from build123d import *

# Parameters (mm, degrees)
F1_DEPTH = 60
F3_D     = 4
F4_D     = 4.5
F5_D     = 5
F6_D     = 5.5
F7_D     = 6
F8_R     = 5.08


with BuildPart() as f1:
    # F0 (on Top) → F1 (new body)
    with BuildSketch(Plane.XY):
        Polygon((-18.362068, 0), (-17.327586, 0), (16.637932, 0), (16.637932, 38.40517), (6.637932, 38.40517), (6.637932, 15), (-8.362068, 15), (-8.362068, 38.40517), (-18.362068, 38.40517), align=None)
    extrude(amount=F1_DEPTH)

    # F3 (through all)
    with Locations(Plane.XZ):
        with Locations((-0.862068, 10)):
            Hole(F3_D / 2)

    # F4 (through all)
    with Locations(Plane.XZ):
        with Locations((-0.862068, 20)):
            Hole(F4_D / 2)

    # F5 (through all)
    with Locations(Plane.XZ):
        with Locations((-0.862068, 30)):
            Hole(F5_D / 2)

    # F6 (through all)
    with Locations(Plane.XZ):
        with Locations((-0.862068, 40)):
            Hole(F6_D / 2)

    # F7 (through all)
    with Locations(Plane.XZ):
        with Locations((-0.862068, 50)):
            Hole(F7_D / 2)

    # F8
    f8_edges = [f1.edges().sort_by_distance(p)[0] for p in [
        (16.637932, 0, 30),
        (-0.862068, 0, 60),
        (-18.362068, 0, 30),
        (-0.862068, 0, 0),
        (-18.362068, 19.202585, 60),
        (16.637932, 19.202585, 60),
        (-18.362068, 19.202585, 0),
        (16.637932, 19.202585, 0),
    ]]
    fillet(f8_edges, radius=F8_R)


solid = f1.part
Part model, mm, in its own coordinate system. A direction names the side the tool comes from. Coordinates: 2 decimals unless noted, no trailing zeros. Order: outer loops, then holes, each group sorted by start corner. A loop starts at its lowest first (then second) coordinate and runs counter-clockwise, first axis right, second up. Notation, with made-up numbers: M -8.75,28 L 22.25,28 A23 ccw 22.25,57 Z; hole C -19,56 d9. An arc over 180 degrees is marked long. One line per question, with ' | ' between items.
Q1. Slice it at A-A (z = 30). Give the cut face in (x, y), and give its area (3 significant figures).
A:
outline: M -18.36,5.08 A5.08 ccw -13.28,0 L -3.36,0 L -3.36,15 L -8.36,15 L -8.36,38.41 L -18.36,38.41 Z; M 1.64,0 L 11.56,0 A5.08 ccw 16.64,5.08 L 16.64,38.41 L 6.64,38.41 L 6.64,15 L 1.64,15 Z | area: 907 mm^2
Q2. Slice it at C-C (x = -0.5). Give the cut face in (y, z), and give its area (3 significant figures).
A:
outline: M 0,5.08 A5.08 ccw 5.08,0 L 15,0 L 15,8.03 L 0,8.03 Z; M 0,11.97 L 15,11.97 L 15,17.78 L 0,17.78 Z; M 0,22.22 L 15,22.22 L 15,27.53 L 0,27.53 Z; M 0,32.47 L 15,32.47 L 15,37.27 L 0,37.27 Z; M 0,42.73 L 15,42.73 L 15,47.02 L 0,47.02 Z; M 0,52.98 L 15,52.98 L 15,60 L 5.08,60 A5.08 ccw 0,54.92 Z | area: 518 mm^2
Q3. Slice it at B-B (y = 28.5). Give the cut face in (x, z), and give its area (3 significant figures).
A:
outline: M -18.36,5.08 A5.08 ccw -13.28,0 L -8.36,0 L -8.36,60 L -13.28,60 A5.08 ccw -18.36,54.92 Z; M 6.64,0 L 11.56,0 A5.08 ccw 16.64,5.08 L 16.64,54.92 A5.08 ccw 11.56,60 L 6.64,60 Z | area: 1,180 mm^2
Q4. Slice it at D-D (y = 13.5). Give the cut face in (x, z).
A:
outline: M -18.36,5.08 A5.08 ccw -13.28,0 L 11.56,0 A5.08 ccw 16.64,5.08 L 16.64,54.92 A5.08 ccw 11.56,60 L -13.28,60 A5.08 ccw -18.36,54.92 Z; hole C -0.86,50 d6; hole C -0.86,40 d5.5; hole C -0.86,30 d5; hole C -0.86,20 d4.5; hole C -0.86,10 d4
Q5. Two-plate mould, pull along Z, no slides. Class faces 3 (the face through (-1, 14.6, 60)), 4 (the face through (-16.913, 21.509, 1.528)), 5 (the face through (-0.504, 7.605, 42.727)): +Z half, -Z half, draft (parallel to the pull), parting line (faces both ways), or undercut.
A:
face 3: +Z half | face 4: -Z half | face 5: undercut
Q6. 3-axis set-ups, long thin cutter, end or side, ignore diameter. For faces 1 (the face through (15.11, 21.98, 58.55)), 2 (the face through (3, 15, 30)): which of +Z, -Z, +X, -X, +Y, -Y reach the whole face in a straight line?
A:
face 1: +Z, +X, +Y, -Y | face 2: +Z, -Z, +Y
Q7. Drill centre lines: line 1 (X direction, y = 16.5, z = 42.5); line 2 (Y direction, x = 6, z = 48); line 3 (X direction, y = 21.5, z = 3). Where is each one in solid material? Low to high.
A:
line 1: x = -18.36 to -8.36, 6.64 to 16.64 | line 2: y = 0 to 15 | line 3: x = -17.92 to -8.36, 6.64 to 16.19
Q8. Pin check, flat tip, straight feed: P1, Ø7.5, axis at x = -1.5, z = 35.5, coming from the +Y side. Stop position of the tip, or through.
A:
P1: stops at y = 15
